Design review of the part built by this model. Coordinates are the model's own, in mm. A direction names the side the tool comes from. Coordinates: 2 decimals unless noted, no trailing zeros. Loops run counter-clockwise (first coordinate to the right, second up) from the corner with the lowest first, then second, coordinate; pieces in that order, holes last. Notation, with made-up numbers: M 42,35 L 86,35 A33 cw 86,67 Z; hole C -15,64.5 d11. An arc over 180 degrees is marked long. Answer as a JSON object with one key per item and string values. Group by question number.
1. Consider section A-A (y = 20). State the section outline as (x, z) points, then the cut area to 3 significant figures.
2. Consider section C-C (x = -19.5). State the section outline as (y, z) points, then the cut area to 3 significant figures.
3. Consider section D-D (z = -17). State the section outline as (x, y) points.
4. To check wall thickness, follow probe 1 along Z at (x, y) = (-16.5, 28); probe 2 along Y at (x, z) = (-68, -167); probe 3 along X at (y, z) = (2, -58). State the ranges of each line that lie inside material, in increasing order.
5. Consider section B-B (z = -110). State the section outline as (x, y) points.
6. Machinability: for faces 1 (the flat face through (-19, 2, -4)), 2 (the flat face through (-34, 16, -178)), 3 (the flat face through (-4, 19, -2)), 4 (the flat face through (-8.5, 2, -178)), 5 (the flat face through (-32, 29, -178)), which of the approach directions +Z, -Z, +X, -X, +Y, -Y give a long, thin tool a straight path to every point of the face, cutting with its end or side? Answer none if there is none.
7. Insertion check: pin 1 (1.2 mm diameter, centred on x = -98, z = -111.5, fed in from -Y); pin 2 (2.5 mm diameter, centred on y = 30, z = -178.5, fed in from +X); pin 3 (1.5 mm diameter, centred on y = 30, z = -178.5, fed in from -X); pin 4 (8 mm diameter, centred on x = -56, y = 9.5, fed in from +Z). Each pin has a flat end and moves straight along its axis. Give the tip position at first contact, or say it passes through.
8. Draft analysis for pull direction X (two halves, no side actions). For faces 6 (the flat face through (0, 4, -91)), 7 (the flat face through (-29.5, 2, -2)), 8 (the flat face through (-98, 32, -91)), state which applies: +X half, -X half, draft (parallel to the pull), parting line (faces both ways), or undercut.
Autodesk Inventor part; units mm, degrees
ref_plane "YZ Plane" through (0, 0, 0) normal (1, 0, 0) x (0, 1, 0)
ref_plane "XZ Plane" through (0, 0, 0) normal (0, 1, 0) x (-1, 0, 0)
ref_plane "XY Plane" through (0, 0, 0) normal (0, 0, 1) x (1, 0, 0)
sketch "Sketch1" plane through (0, 0, 0) normal (0, 1, 0) x (-1, 0, 0)
  line L0 (0, 0) -> (100, 0)
  line L1 (100, 0) -> (100, -180)
  line L2 (100, -180) -> (0, -180)
  line L3 (0, -180) -> (0, 0)
  dimension "d0" = 100
  dimension "d1" = 180
extrude "Extrusion1" add sketch "Sketch1" along normal blind 4
sketch "Sketch2" plane through (0, 4, 0) normal (0, 1, 0) x (1, 0, 0)
  line L0 (-100, 180) -> (-100, 0)
  line L1 (0, 180) -> (-100, 180)
  line L2 (-100, 0) -> (-96, 0)
  line L3 (-96, 0) -> (-96, 180)
  line L4 (-96, 180) -> (-100, 180)
  line L5 (-100, 180) -> (-100, 0)
  line L6 (0, 180) -> (-4, 180)
  line L7 (-4, 180) -> (-4, 0)
  line L8 (-4, 0) -> (0, 0)
  line L9 (0, 0) -> (0, 180)
  dimension "d4" = 4
  dimension "d5" = 4
extrude "Extrusion2" add sketch "Sketch2" along normal blind 5 contours L1 L9 L8 L7
sketch "Sketch3" plane through (0, 4, 0) normal (0, 1, 0) x (1, 0, 0)
  line L0 (-4, 180) -> (-4, 0)
  line L1 (-4, 0) -> (-34, 0)
  line L2 (-34, 0) -> (-34, 4)
  line L3 (-34, 4) -> (-4, 4)
  line L4 (-4, 4) -> (-4, 0)
  line L5 (-4, 180) -> (-100, 180)
  line L6 (-4, 180) -> (-34, 180)
  line L7 (-34, 180) -> (-34, 176)
  line L8 (-34, 176) -> (-4, 176)
  line L9 (-4, 176) -> (-4, 180)
  line L10 (-100, 0) -> (0, 0)
  line L11 (-100, 0) -> (-96, 0)
  line L12 (-96, 0) -> (-96, 180)
  line L13 (-96, 180) -> (-100, 180)
  line L14 (-100, 180) -> (-100, 0)
  point P0 (-4, 176)
  point P1 (-4, 4)
  dimension "d8" = 30
  dimension "d9" = 4
  dimension "d10" = 4
  dimension "d11" = 4
extrude "Extrusion3" add sketch "Sketch3" along normal blind 25 contours L0 L8 L7 L5 | L0 L1 L2 L3 | L12 L10 L14 L5
sketch "Sketch4" plane through (0, 29, 0) normal (0, 1, 0) x (1, 0, 0)
  line L0 (-100, 0) -> (-96, 0)
  line L1 (-96, 0) -> (-96, 180)
  line L2 (-96, 180) -> (-100, 180)
  line L3 (-100, 180) -> (-100, 0)
  line L4 (-4, 176) -> (-4, 180)
  line L5 (-4, 180) -> (-34, 180)
  line L6 (-34, 180) -> (-34, 176)
  line L7 (-34, 176) -> (-4, 176)
  line L8 (-34, 0) -> (-4, 0)
  line L9 (-34, 4) -> (-34, 0)
  line L10 (-34, 0) -> (-4, 0)
  line L11 (-4, 0) -> (-4, 4)
  line L12 (-4, 4) -> (-34, 4)
  line L13 (-100, 90) -> (-100, 145)
  line L14 (-100, 145) -> (-96, 145)
  line L15 (-96, 145) -> (-96, 35)
  line L16 (-96, 0) -> (-96, 180)
  line L17 (-96, 35) -> (-100, 35)
  line L18 (-100, 35) -> (-100, 90)
  line L19 (-4, 176) -> (-34, 176)
  line L20 (-19, 176) -> (-29, 176)
  line L21 (-29, 176) -> (-29, 180)
  line L22 (-29, 180) -> (-9, 180)
  line L23 (0, 180) -> (-100, 180)
  line L24 (-9, 180) -> (-9, 176)
  line L25 (-19, 176) -> (-9, 176)
  line L26 (-19, 4) -> (-29, 4)
  line L27 (-29, 4) -> (-29, 0)
  line L28 (-29, 0) -> (-9, 0)
  line L29 (-9, 0) -> (-9, 4)
  line L30 (-4, 4) -> (-34, 4)
  line L31 (-9, 4) -> (-19, 4)
  point P0 (0, 0)
  dimension "d14" = 55
  dimension "d15" = 110
  dimension "d16" = 10
  dimension "d17" = 20
extrude "Extrusion4" add sketch "Sketch4" along normal blind 3 contours L3 L14 L1 L17 | L5 L24 L7 L21 | L27 L12 L29 L8
sketch "Sketch5" plane through (0, 0, 0) normal (0, -1, 0) x (1, 0, 0)
  line L0 (-9, -4) -> (-29, -4)
  line L1 (-29, -4) -> (-29, 0)
  line L2 (-29, 0) -> (-9, 0)
  line L3 (-9, 0) -> (-9, -4)
  line L4 (-9, -180) -> (-29, -180)
  line L5 (-29, -180) -> (-29, -176)
  line L6 (-29, -176) -> (-9, -176)
  line L7 (-9, -176) -> (-9, -180)
  line L8 (-96, -35) -> (-96, -145)
  line L9 (-96, -145) -> (-100, -145)
  line L10 (-100, -145) -> (-100, -35)
  line L11 (-100, -35) -> (-96, -35)
  line L12 (-96, -180) -> (-96, 0)
  line L13 (-100, -35) -> (-96, -35)
  line L14 (-96, -35) -> (-96, -34.5)
  line L15 (-96, -34.5) -> (-100, -34.5)
  line L16 (-100, -34.5) -> (-100, -35)
  line L17 (-100, -145) -> (-96, -145)
  line L18 (-96, -145) -> (-96, -145.5)
  line L19 (-96, -145.5) -> (-100, -145.5)
  line L20 (-100, -145.5) -> (-100, -145)
  line L21 (-4, -176) -> (-34, -176)
  line L22 (-29, -180) -> (-29.5, -180)
  line L23 (-29.5, -180) -> (-29.5, -176)
  line L24 (-29.5, -176) -> (-29, -176)
  line L25 (-29, -176) -> (-29, -180)
  line L26 (-9, -176) -> (-8.5, -176)
  line L27 (-8.5, -176) -> (-8.5, -180)
  line L28 (-8.5, -180) -> (-9, -180)
  line L29 (-9, -180) -> (-9, -176)
  line L30 (-34, -4) -> (-4, -4)
  line L31 (-29, 0) -> (-29.5, 0)
  line L32 (-29.5, 0) -> (-29.5, -4)
  line L33 (-29.5, -4) -> (-29, -4)
  line L34 (-29, -4) -> (-29, 0)
  line L35 (-9, 0) -> (-8.5, 0)
  line L36 (-8.5, 0) -> (-8.5, -4)
  line L37 (-8.5, -4) -> (-9, -4)
  line L38 (-9, -4) -> (-9, 0)
  point P0 (0, 0)
  dimension "d22" = 0.5
  dimension "d23" = 0.5
  dimension "d24" = 0.5
  dimension "d25" = 0.5
  dimension "d26" = 0.5
  dimension "d27" = 0.5
extrude "Extrusion5" cut sketch "Sketch5" against normal blind 3.2
properties part number "caja_attiny"
Findings below:
{
 "1": {"outline": "M -100,-180 L -96,-180 L -96,0 L -100,0 Z; M -34,-180 L -4,-180 L -4,-176 L -34,-176 Z; M -34,-4 L -4,-4 L -4,0 L -34,0 Z", "area": "960 mm^2"},
 "2": {"outline": "M 0,-176 L 3.2,-176 L 3.2,-180 L 32,-180 L 32,-176 L 4,-176 L 4,-4 L 32,-4 L 32,0 L 3.2,0 L 3.2,-4 L 0,-4 Z", "area": "918 mm^2"},
 "3": {"outline": "M -100,0 L 0,0 L 0,9 L -4,9 L -4,4 L -96,4 L -96,29 L -100,29 Z"},
 "4": {"probe 1": "z = -180 to -176, -4 to 0", "probe 2": "y = 0 to 4", "probe 3": "x = -96 to 0"},
 "5": {"outline": "M -100,3.2 L -96,3.2 L -96,0 L 0,0 L 0,9 L -4,9 L -4,4 L -96,4 L -96,32 L -100,32 Z"},
 "6": {"face 1": "+Z, -Y", "face 2": "+Z, -Z, +Y", "face 3": "+Z, -Z, +X, +Y", "face 4": "-Z, -Y", "face 5": "+Z, -Z, -X, +Y"},
 "7": {"pin 1": "stops at y = 3.2", "pin 2": "stops at x = -4", "pin 3": "stops at x = -29", "pin 4": "passes through"},
 "8": {"face 6": "+X half", "face 7": "undercut", "face 8": "draft"}
}
